Part model, mm, in its own coordinate system. Face numbers are marked on the shaded views. A direction names the side the tool comes from. Round coordinates to 2 decimals unless told otherwise and drop trailing zeros. Use CSV: the item, a comma, the result in double quotes. Start each with the question number.
(1) Which spindle directions (+Z, -Z, +X, -X, +Y, -Y) get a long thin tool onto all of the face, cutting with end or side? Do the marked faces 4, 5 and 6. Say none if no direction does.
(2) Drop flat-ended pins along their axis: pin 1 (1.5 mm diameter, centred on x = 0.5, z = -6.5, fed in from +Y); pin 2 (1.5 mm diameter, centred on y = 6, z = -5.5, fed in from -X); pin 3 (4 mm diameter, centred on y = -6.5, z = 0, fed in from +X); pin 4 (11 mm diameter, centred on x = -1.5, y = -1.5, fed in from -Z). Give the stop position or say it passes through.
(3) Two-plate mould, pull along X, no slides. Class the marked faces 1, 2 and 3: released by +X, released by -X, zero draft, split by the parting line, or undercut.
(4) Probe line 1 (Z direction, x = 16.5, y = -4.5); line 2 (Y direction, x = 7, z = -1.25); line 3 (Y direction, x = 3, z = -1). List the from-to ranges inside material, lowest first. Write a range as [from, to].
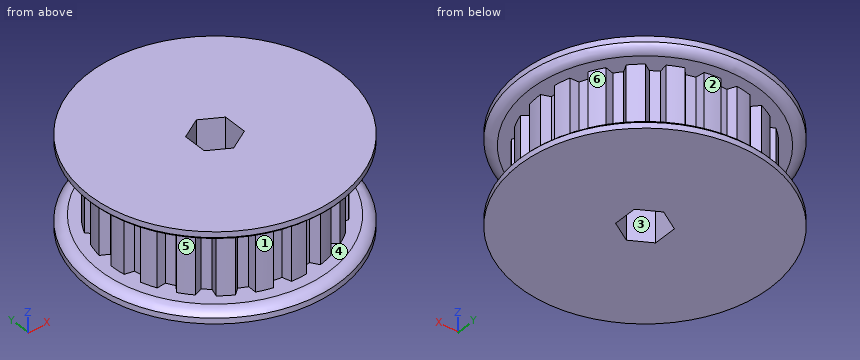
```python
from build123d import *

# Parameters (mm, degrees)
CUT_EXTRUDE1_START = 1.397
CUT_EXTRUDE1_DEPTH = 10.7188
CIRPATTERN1_COUNT  = 21
SKETCH4_R          = 1.5875
CUT_EXTRUDE2_DEPTH = 31.241836167
CUT_EXTRUDE3_DEPTH = 1.190625
CIRPATTERN2_COUNT  = 2
CIRPATTERN2_ANGLE  = 90
CUT_EXTRUDE4_DEPTH = 50.8
SKETCH8_R          = 12.7
CUT_EXTRUDE5_DEPTH = 50.8


with BuildPart() as part:
    # Sketch2 → Revolve1 (revolve)
    with BuildSketch(Plane(origin=(0, 0, 0), x_dir=(0, 0, -1), z_dir=(1, 0, 0)), mode=Mode.PRIVATE) as revolve1_sk:
        with BuildLine():
            Line((-11.1125, 3.175), (11.1125, 3.175))
            Line((11.1125, 3.175), (11.1125, 19.8882))
            Line((11.1125, 19.8882), (10.21715, 19.8882))
            ThreePointArc((10.21715, 19.8882), (9.559562343, 19.158250378), (9.3218, 18.204983865))
            Line((9.3218, 18.204983865), (9.3218, 16.521767729))
            Line((9.3218, 16.521767729), (-1.397, 16.521767729))
            Line((-1.397, 16.521767729), (-1.397, 18.204983865))
            ThreePointArc((-1.397, 18.204983865), (-1.634762343, 19.158250378), (-2.29235, 19.8882))
            Line((-2.29235, 19.8882), (-3.1877, 19.8882))
            Line((-3.1877, 19.8882), (-3.1877, 11.9126))
            Line((-3.1877, 11.9126), (-11.1125, 11.9126))
            Line((-11.1125, 11.9126), (-11.1125, 3.175))
        make_face()
    revolve(revolve1_sk.sketch.rotate(Axis((0, 0, 11.1125), (0, 0, -1)), 90), axis=Axis((0, 0, 11.1125), (0, 0, -1)))

    # Sketch3 → Cut-Extrude1 (cut)
    with BuildSketch(Plane.XY.offset(CUT_EXTRUDE1_START)):
        with BuildLine():
            Line((-0.690489274, 15.2019), (0.690489274, 15.2019))
            Line((0.690489274, 15.2019), (1.2827, 16.4719))
            ThreePointArc((1.2827, 16.4719), (0, 16.521767729), (-1.2827, 16.4719))
            Line((-1.2827, 16.4719), (-0.690489274, 15.2019))
        make_face()
    cut_extrude1 = extrude(amount=-CUT_EXTRUDE1_DEPTH, mode=Mode.SUBTRACT)

    # CirPattern1: Cut-Extrude1 ×21 about axis
    cirpattern1_axis = Axis((0, 0, 0), (0, 0, 1))
    for i in range(1, CIRPATTERN1_COUNT):
        add(cut_extrude1.rotate(cirpattern1_axis, i * 360 / CIRPATTERN1_COUNT), mode=Mode.SUBTRACT)

    # Sketch4 → Cut-Extrude2 (cut, through all)
    with BuildSketch(Plane(origin=(0, 0, 0), x_dir=(1, 0, 0), z_dir=(0, 1, 0))):
        with Locations(Location((0, -7.1501, 0), (0, 0, 90))):
            Circle(SKETCH4_R)
    cut_extrude2 = extrude(amount=CUT_EXTRUDE2_DEPTH, mode=Mode.SUBTRACT)

    # Sketch5 → Revolve2 (revolve)
    with BuildSketch(Plane.XY.offset(7.1501), mode=Mode.PRIVATE) as revolve2_sk:
        Polygon((1.0795, 11.806349246), (1.5875, 11.298349246), (1.5875, 3.81), (0.9525, 3.175), (0, 3.175), (0, 11.806349246), align=None)
    revolve2 = revolve(revolve2_sk.sketch.rotate(Axis((0, 0, 7.1501), (0, 1, 0)), 90), axis=Axis((0, 0, 7.1501), (0, 1, 0)))

    # Sketch6 → Cut-Extrude3 (cut)
    with BuildSketch(Plane(origin=(0, 11.806349246, 0), x_dir=(1, 0, 0), z_dir=(0, 1, 0))):
        Polygon((0, -6.233556448), (-0.79375, -6.691828224), (-0.79375, -7.608371776), (0, -8.066643552), (0.79375, -7.608371776), (0.79375, -6.691828224), align=None)
    cut_extrude3 = extrude(amount=-CUT_EXTRUDE3_DEPTH, mode=Mode.SUBTRACT)

    # CirPattern2: Cut-Extrude2, Revolve2, Cut-Extrude3 ×2 about axis
    cirpattern2_axis = Axis((0, 0, 0), (0, 0, -1))
    add([cut_extrude2.rotate(cirpattern2_axis, i * CIRPATTERN2_ANGLE / (CIRPATTERN2_COUNT - 1)) for i in range(1, CIRPATTERN2_COUNT)], mode=Mode.SUBTRACT)
    add([revolve2.rotate(cirpattern2_axis, i * CIRPATTERN2_ANGLE / (CIRPATTERN2_COUNT - 1)) for i in range(1, CIRPATTERN2_COUNT)])
    add([cut_extrude3.rotate(cirpattern2_axis, i * CIRPATTERN2_ANGLE / (CIRPATTERN2_COUNT - 1)) for i in range(1, CIRPATTERN2_COUNT)], mode=Mode.SUBTRACT)

    # Sketch7 → Cut-Extrude4 (cut)
    with BuildSketch(Plane.XY.offset(11.1125)):
        Polygon((0, 3.666174209), (-3.175, 1.833087105), (-3.175, -1.833087105), (0, -3.666174209), (3.175, -1.833087105), (3.175, 1.833087105), align=None)
    extrude(amount=-CUT_EXTRUDE4_DEPTH, mode=Mode.SUBTRACT)

    # Sketch8 → Cut-Extrude5 (cut)
    with BuildSketch(Plane.XY.offset(3.1877)):
        Circle(SKETCH8_R)
    extrude(amount=CUT_EXTRUDE5_DEPTH, mode=Mode.SUBTRACT)


solid = part.part
```
Answers:
1,face 4,"none"
1,face 5,"-X, -Y"
1,face 6,"+X, +Y"
2,pin 1,"stops at y = 16.4"
2,pin 2,"stops at x = -14.43"
2,pin 3,"stops at x = 18.64"
2,pin 4,"stops at z = -11.11"
3,face 1,"released by -X"
3,face 2,"released by +X"
3,face 3,"undercut"
4,line 1,"z = [-11.11, -9.32], [1.4, 3.19]"
4,line 2,"y = [-13.5, 14.97]"
4,line 3,"y = [-15.01, -1.93], [1.93, 16.25]"
